```python
from build123d import *

# Parameters (mm, degrees)
SKETCH1_R           = 137.5
SKETCH1_R_2         = 125
BOSS_EXTRUDE1_DEPTH = 180
SKETCH2_R           = 157.5
BOSS_EXTRUDE2_DEPTH = 10
SKETCH3_R           = 52.5
SKETCH3_R_2         = 47.5
BOSS_EXTRUDE3_DEPTH = 20
SKETCH4_W           = 56
SKETCH4_H           = 96
CUT_EXTRUDE4_DEPTH  = 150
SKETCH5_W           = 56
SKETCH5_H           = 10
BOSS_EXTRUDE4_DEPTH = 56
SKETCH6_W           = 56
SKETCH6_H           = 56
BOSS_EXTRUDE5_DEPTH = 10
SKETCH7_R           = 2.5
SKETCH7_R_2         = 12.5
CUT_EXTRUDE5_DEPTH  = 10
SKETCH8_W           = 56
SKETCH8_H           = 86
BOSS_EXTRUDE6_DEPTH = 5
FILLET1_R           = 10
FILLET2_R           = 5
SKETCH9_W           = 31.730677801
SKETCH9_H           = 6
CUT_EXTRUDE6_DEPTH  = 10
FILLET3_R           = 5
CUT_EXTRUDE7_START  = -2
SKETCH10_R          = 47.5
CUT_EXTRUDE7_DEPTH  = 2


with BuildPart() as part:
    # Sketch1 → Boss-Extrude1 (new body)
    with BuildSketch(Plane(origin=(0, 0, 0), x_dir=(1, 0, 0), z_dir=(0, 1, 0))):
        with Locations(Location((0, 0, 0), (0, 0, 90))):
            Circle(SKETCH1_R)
        with Locations(Location((0, 0, 0), (0, 0, 90))):
            Circle(SKETCH1_R_2, mode=Mode.SUBTRACT)
    extrude(amount=BOSS_EXTRUDE1_DEPTH)

    # Sketch2 → Boss-Extrude2 (add)
    with BuildSketch(Plane.XZ):
        with Locations(Location((0, 0, 0), (0, 0, 270))):
            Circle(SKETCH2_R)
    extrude(amount=BOSS_EXTRUDE2_DEPTH)

    # Sketch3 → Boss-Extrude3 (add)
    with BuildSketch(Plane(origin=(0, 0, 0), x_dir=(1, 0, 0), z_dir=(0, 1, 0))):
        with Locations(Location((0, 0, 0), (0, 0, 90))):
            Circle(SKETCH3_R)
        with Locations(Location((0, 0, 0), (0, 0, 270))):
            Circle(SKETCH3_R_2, mode=Mode.SUBTRACT)
    extrude(amount=BOSS_EXTRUDE3_DEPTH)

    # Sketch4 → Cut-Extrude4 (cut)
    with BuildSketch(Plane(origin=(0, 0, 0), x_dir=(0, 0, -1), z_dir=(1, 0, 0))):
        with Locations((0, 112)):
            Rectangle(SKETCH4_W, SKETCH4_H)
    extrude(amount=CUT_EXTRUDE4_DEPTH, mode=Mode.SUBTRACT)

    # Sketch5 → Boss-Extrude4 (add)
    with BuildSketch(Plane(origin=(0, 0, 28), x_dir=(-1, 0, 0), z_dir=(0, 0, -1))):
        with Locations((-121.823643025, 135)):
            Rectangle(SKETCH5_W, SKETCH5_H)
    extrude(amount=BOSS_EXTRUDE4_DEPTH)

    # Sketch6 → Boss-Extrude5 (add)
    with BuildSketch(Plane(origin=(0, 64, 0), x_dir=(1, 0, 0), z_dir=(0, 1, 0))):
        with Locations((121.823643025, 0)):
            Rectangle(SKETCH6_W, SKETCH6_H)
    extrude(amount=-BOSS_EXTRUDE5_DEPTH)

    # Sketch7 → Cut-Extrude5 (cut)
    with BuildSketch(Plane(origin=(0, 140, 0), x_dir=(1, 0, 0), z_dir=(0, 1, 0))):
        with Locations(Location((98.273643025, 23.55, 0), (0, 0, 270))):
            Circle(SKETCH7_R)
        with Locations(Location((145.373643025, 23.55, 0), (0, 0, 270))):
            Circle(SKETCH7_R)
        with Locations(Location((98.273643025, -23.55, 0), (0, 0, 270))):
            Circle(SKETCH7_R)
        with Locations(Location((145.373643025, -23.55, 0), (0, 0, 270))):
            Circle(SKETCH7_R)
        with Locations(Location((121.823643025, 0, 0), (0, 0, 270))):
            Circle(SKETCH7_R_2)
    extrude(amount=-CUT_EXTRUDE5_DEPTH, mode=Mode.SUBTRACT)

    # Sketch8 → Boss-Extrude6 (add)
    with BuildSketch(Plane(origin=(149.823643025, 0, 0), x_dir=(0, 0, -1), z_dir=(1, 0, 0))):
        with Locations((0, 97)):
            Rectangle(SKETCH8_W, SKETCH8_H)
    extrude(amount=BOSS_EXTRUDE6_DEPTH)

    # Fillet1
    # the kernel refuses this fillet: 10 mm, written as the material it takes off along each edge
    with BuildSketch(Plane(origin=(154.823643025, 165, -28), x_dir=(0, 0, 1), z_dir=(0, -1, 0)), Plane(origin=(154.823643025, 29, 28), x_dir=(0, 0, -1), z_dir=(0, 1, 0))) as fillet1_piece_1:
        with BuildLine():
            CenterArc((FILLET1_R, FILLET1_R), FILLET1_R, 180, 90)
            Line((0, FILLET1_R), (0, 0))
            Line((0, 0), (FILLET1_R, 0))
        make_face()
    extrude(amount=136, mode=Mode.SUBTRACT)

    # Fillet2
    fillet2_edges = [part.edges().sort_by_distance(p)[0] for p in [
        (93.823643025, 135, -28),
        (93.823643025, 135, 28),
        (93.823643025, 59, 28),
        (93.823643025, 59, -28),
    ]]
    fillet(fillet2_edges, radius=FILLET2_R)

    # Sketch9 → Cut-Extrude6 (cut)
    with BuildSketch(Plane(origin=(0, 140, 0), x_dir=(1, 0, 0), z_dir=(0, 1, 0))):
        with Locations((93.823643026, 0)):
            Rectangle(SKETCH9_W, SKETCH9_H)
    extrude(amount=-CUT_EXTRUDE6_DEPTH, mode=Mode.SUBTRACT)

    # Fillet3
    fillet3_edges = [part.edges().sort_by_distance(p)[0] for p in [
        (0, 180, 137.5),
    ]]
    fillet(fillet3_edges, radius=FILLET3_R)

    # Sketch10 → Cut-Extrude7 (cut)
    with BuildSketch(Plane(origin=(0, 0, 0), x_dir=(1, 0, 0), z_dir=(0, 1, 0)).offset(CUT_EXTRUDE7_START)):
        with Locations(Location((0, 0, 0), (0, 0, 270))):
            Circle(SKETCH10_R)
    extrude(amount=CUT_EXTRUDE7_DEPTH, mode=Mode.SUBTRACT)


solid = part.part
```
Build history of the part. All positions in model axes, mm. A direction names the side the tool comes from. Give positions to 0.01 mm unless a question says otherwise; leave off trailing zeros. Loops run counter-clockwise (first coordinate to the right, second up) from the corner with the lowest first, then second, coordinate; pieces in that order, holes last.
Item 1: Flat gauge pins, fed straight in: pin 1 (11 mm diameter, centred on x = 142, y = 59.5, fed in from +Z); pin 2 (6 mm diameter, centred on x = -79.5, y = 17, fed in from -Z); pin 3 (5 mm diameter, centred on x = 15, y = 137.5, fed in from -Z). Where does each tip first touch, or does it go through?
Answers follow:
pin 1: stops at z = 28
pin 2: stops at z = -114.25
pin 3: stops at z = -136.93
Item 2: Pull direction Z, two halves, no side cores. Call faces 5 (the face through (110, 135, 28)), 6 (the face through (152.95, 97.6, -23.83)), 7 (the face through (145, 54, 0)): released by +Z, released by -Z, zero draft, split by the parting line, or undercut.
Answers follow:
face 5: undercut
face 6: released by -Z
face 7: zero draft
Item 3: Slice it at A-A, the plane x = 0. List the corners of the cut face in (y, z).
Answers follow:
outline: (-10, -157.5) - (0, -157.5) - (0, -137.5) - (175, -137.5) arc R5 ccw to (180, -132.5) - (180, -125) - (0, -125) - (0, -52.5) - (20, -52.5) - (20, -47.5) - (-2, -47.5) - (-2, 47.5) - (20, 47.5) - (20, 52.5) - (0, 52.5) - (0, 125) - (180, 125) - (180, 132.5) arc R5 ccw to (175, 137.5) - (0, 137.5) - (0, 157.5) - (-10, 157.5) - close
Item 4: Drill centre lines: line 1 (X direction, y = 135, z = 0); line 2 (X direction, y = 136.5, z = -23.55); line 3 (Z direction, x = -2, y = 120). Where is each one in solid material? Low to high.
Answers follow:
line 1: x = -137.5 to -125, 134.32 to 154.82
line 2: x = -135.47 to -122.76, 93.85 to 95.77, 100.77 to 142.87, 147.87 to 153.14
line 3: z = -137.49 to -124.98, 124.98 to 137.49
Item 5: Slice it at B-B, the plane y = 153.5. List the corners of the cut face in (x, z), and give its area (3 significant figures).
Answers follow:
outline: (121.82, -28) arc R125 cw (long way) to (121.82, 28) - (134.62, 28) arc R137.5 ccw (long way) to (134.62, -28) - close
area: 9,600 mm2
Item 6: Which spindle directions (+Z, -Z, +X, -X, +Y, -Y) get a long thin tool onto all of the face, cutting with end or side? Do faces 1 (the face through (2, -10, 2)), 2 (the face through (46.4, 20, 11.9)), 3 (the face through (121, 64, 0)), 4 (the face through (140, 135, 28)). Say none if no direction does.
Answers follow:
face 1: +Z, -Z, +X, -X, -Y
face 2: +Y
face 3: none
face 4: +Z, +X, +Y
